Can you work these out from the model? Positions are in its coordinate system, mm. Coordinates: 2 decimals unless noted, no trailing zeros. Write each loop counter-clockwise with the first axis right and the second up, starting at its lowest first coordinate (ties: lowest second). Pieces come first, ordered by that corner, then holes. Notation, with made-up numbers: M 29,-36 L 65,-36 A14 ccw 65,-12 Z; hole C -9,-27.5 d2. An arc over 180 degrees is marked long. Answer as a JSON object with one key per item and string values. Group by question number.
Autodesk Inventor part; units mm, degrees
ref_plane "YZ Plane" through (0, 0, 0) normal (1, 0, 0) x (0, 1, 0)
ref_plane "XZ Plane" through (0, 0, 0) normal (0, 1, 0) x (-1, 0, 0)
ref_plane "XY Plane" through (0, 0, 0) normal (0, 0, 1) x (1, 0, 0)
sketch "Szkic1" plane through (0, 0, 0) normal (0, 0, 1) x (1, 0, 0)
  line L0 (0, 0) -> (80, 0)
  line L1 (80, 0) -> (80, 80)
  line L2 (80, 80) -> (0, 80)
  line L3 (0, 80) -> (0, 0)
  dimension "d0" = 80
  dimension "d1" = 80
extrude "Wyciągnięcie proste1" add sketch "Szkic1" along normal blind 5
sketch "Szkic2" plane through (0, 0, 5) normal (0, 0, 1) x (1, 0, 0)
  line L0 (80, 0) -> (80, 80)
  line L1 (80, 0) -> (39, 0)
  line L2 (39, 0) -> (39, 5)
  line L3 (39, 5) -> (80, 5)
  line L4 (80, 5) -> (80, 0)
  point P0 (0, 0)
  dimension "d6" = 41
  dimension "d7" = 5
extrude "Wyciągnięcie proste2" add sketch "Szkic2" along normal blind 41
sketch "Szkic3" plane through (0, 0, 5) normal (0, 0, 1) x (1, 0, 0)
  line L0 (19, 35.2968) -> (24, 35.2968)
  line L1 (24, 35.2968) -> (24, 30.2968)
  line L2 (24, 30.2968) -> (19, 30.2968)
  line L3 (19, 30.2968) -> (19, 35.2968)
  line L4 (19, 15.2968) -> (24, 15.2968)
  line L5 (24, 15.2968) -> (24, 10.2968)
  line L6 (24, 10.2968) -> (19, 10.2968)
  line L7 (19, 10.2968) -> (19, 15.2968)
  line L8 (39, 5) -> (39, 0)
  point P0 (0, 0)
  point P1 (39, 2.5)
  point P2 (24, 12.7968)
  dimension "d10" = 5
  dimension "d11" = 5
  dimension "d12" = 5
  dimension "d13" = 15
  dimension "d14" = 15
extrude "Wyciągnięcie proste3" add sketch "Szkic3" along normal blind 10
sketch "Szkic4" plane through (0, 0, 5) normal (0, 0, 1) x (1, 0, 0)
  line L0 (80, 80) -> (0, 80)
  line L1 (80, 5) -> (80, 80)
  point P0 (0, 0)
  point P1 (32.5, 68.05)
  point P2 (47.5, 68.05)
  point P3 (47.5, 52.05)
  point P4 (32.5, 52.05)
  dimension "d17" = 11.95
  dimension "d18" = 11.95
  dimension "d19" = 15
  dimension "d20" = 15
  dimension "d21" = 16
  dimension "d22" = 16
  dimension "d23" = 32.5
  dimension "d24" = 32.5
hole "Otwór1" at (32.5, 68.05, 5) at (47.5, 68.05, 5) at (47.5, 52.05, 5) at (32.5, 52.05, 5) direction (0, 0, -1) diameter 2.5 depth 5 countersink diameter 4.4 countersink angle 90
sketch "Szkic5" plane through (39, 0, 5) normal (-1, 0, 0) x (0, 0, 1)
  line L0 (-5, 0) -> (41, 0)
  line L1 (21, 0) -> (25, 0)
  line L2 (25, 0) -> (25, 35)
  line L3 (25, 35) -> (21, 35)
  line L4 (21, 35) -> (21, 0)
  line L5 (0, 80) -> (0, 0)
  dimension "d32" = 4
  dimension "d33" = 35
  dimension "d34" = 21
extrude "Wyciągnięcie proste4" add sketch "Szkic5" along normal blind 7
sketch "Szkic6" plane through (80, 0, 0) normal (1, 0, 0) x (0, 0, -1)
  line L0 (-30, 5) -> (-30, 35)
  line L1 (-5, 0) -> (-26, 0)
  line L2 (-30, 35) -> (-26, 35)
  line L3 (-26, 35) -> (-26, 0)
  line L4 (-26, 0) -> (-30, 0)
  line L5 (-30, 0) -> (-30, 35)
  point P0 (0, 0)
  point P1 (-30, 5)
extrude "Wyciągnięcie proste5" add sketch "Szkic6" along normal blind 7
sketch "Szkic10" plane through (39, 5, 30) normal (0, 0, 1) x (1, 0, 0)
  line L0 (0, -5) -> (-7, -5)
  line L1 (41, -5) -> (48, -5)
  line L2 (-7, -5) -> (-7, 30)
  line L3 (48, 30) -> (48, -5)
  point P0 (-39, -5)
  point P1 (-4.25, 15)
  point P2 (-4.25, 5)
  point P3 (45.25, 15)
  point P4 (45.25, 5)
  point P5 (-3.5, -5)
  dimension "d43" = 10
  dimension "d46" = 10
  dimension "d47" = 10
  dimension "d48" = 2.75
  dimension "d49" = 2.75
  dimension "d50" = 10
  dimension "d51" = 2.75
  dimension "d52" = 2.75
hole "Otwór2" at (34.75, 20, 30) at (34.75, 10, 30) at (84.25, 20, 30) at (84.25, 10, 30) direction (0, 0, -1) diameter 4.5 depth 4
properties part number "podstawa_rysika"
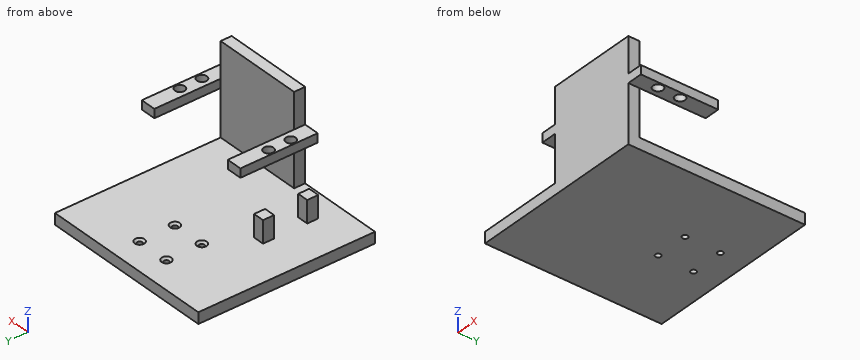
Q1. If we section it at C-C on y = 52.05: List the corners of the cut face in (x, z) for me, and give its area (3 significant figures).
Q2. If we section it at D-D on z = 10: List the corners of the cut face in (x, y) for me.
Q3. If we section it at B-B on z = 28: List the corners of the cut face in (x, y) for me.
Q4. If we section it at A-A on x = 84.25: List the corners of the cut face in (y, z) for me, and give its area (3 significant figures).
Q5. Please list where these lines run through material, in increasing order: L1, parallel to X at y = 10, z = 27; L2, parallel to Y at x = 47.5, z = 1.4; L3, parallel to Y at x = 34.75, z = 27.95.
Q6. Will these pins go through, and if not, where does the flat tip stop? pin 1 (10 mm diameter, centred on y = 17, z = 17.5, fed in from +X); pin 2 (5.5 mm diameter, centred on y = 3.5, z = 14.5, fed in from -X); pin 3 (10 mm diameter, centred on x = 78, y = 57, fed in from +Z); pin 4 (1.5 mm diameter, centred on x = 32.5, y = 52.05, fed in from -Z).
Reply:
{
 "1": {"outline": "M 0,0 L 31.25,0 L 31.25,4.05 L 30.3,5 L 0,5 Z; M 33.75,0 L 46.25,0 L 46.25,4.05 L 45.3,5 L 34.7,5 L 33.75,4.05 Z; M 48.75,0 L 80,0 L 80,5 L 49.7,5 L 48.75,4.05 Z", "area": "373 mm^2"},
 "2": {"outline": "M 19,10.3 L 24,10.3 L 24,15.3 L 19,15.3 Z; M 19,30.3 L 24,30.3 L 24,35.3 L 19,35.3 Z; M 39,0 L 80,0 L 80,5 L 39,5 Z"},
 "3": {"outline": "M 32,0 L 87,0 L 87,35 L 80,35 L 80,5 L 39,5 L 39,35 L 32,35 Z; hole C 34.75,10 d4.5; hole C 34.75,20 d4.5; hole C 84.25,10 d4.5; hole C 84.25,20 d4.5"},
 "4": {"outline": "M 0,26 L 7.75,26 L 7.75,30 L 0,30 Z; M 12.25,26 L 17.75,26 L 17.75,30 L 12.25,30 Z; M 22.25,26 L 35,26 L 35,30 L 22.25,30 Z", "area": "104 mm^2"},
 "5": {"L1": "32 to 32.5, 37 to 39, 80 to 82, 86.5 to 87", "L2": "0 to 50.8, 53.3 to 66.8, 69.3 to 80", "L3": "0 to 7.75, 12.25 to 17.75, 22.25 to 35"},
 "6": {"pin 1": "x = 24", "pin 2": "x = 39", "pin 3": "z = 5", "pin 4": "through"}
}
